Autodesk Inventor part; units mm, degrees
ref_plane "YZ Plane" through (0, 0, 0) normal (1, 0, 0) x (0, 1, 0)
ref_plane "XZ Plane" through (0, 0, 0) normal (0, 1, 0) x (-1, 0, 0)
ref_plane "XY Plane" through (0, 0, 0) normal (0, 0, 1) x (1, 0, 0)
sketch "Эскиз1" plane through (0, 0, 0) normal (0, 0, 1) x (1, 0, 0)
  line L0 (0, 81) -> (0, 93)
  line L1 (0, 93) -> (-11, 93)
  line L2 (-11, 93) -> (-11, 81.2677)
  line L3 (-11, 81.2677) -> (-42, 50)
  line L4 (-42, 50) -> (-42, 26)
  line L5 (-42, 26) -> (-38, 26)
  line L6 (-38, 26) -> (-38, 42.6719)
  line L7 (-38, 42.6719) -> (0, 81)
  line L8 (0, 0) -> (0, 108.7974) construction
  line L9 (-50.4, 0) -> (8.4, 0)
  dimension "d0" = 11
  dimension "d1" = 12
  dimension "d2" = 24
  dimension "d3" = 4
  dimension "d4" = 8
  dimension "d5" = 67
  dimension "d6" = 42
  dimension "d7" = 93
revolve "Вращение1" add sketch "Эскиз1" angle 360 about axis through (-10, 0, 0) along (1, 0, 0)
hole "Отверстие1" at (-11, -0.0233, 87.0155) direction (1, 0, 0) diameter 5 end through all counterbore diameter 9 counterbore depth 5
pattern_circular "Круговой массив1" count 6 over 360 about axis through (-10, 0, 0) along (1, 0, 0) of "Отверстие1"
CAD build for the part. Positions are in the model's coordinates, mm. A direction names the side the tool comes from. Round coordinates to 2 decimals unless told otherwise and drop trailing zeros. Write each loop counter-clockwise with the first axis right and the second up, starting at its lowest first coordinate (ties: lowest second). Pieces come first, ordered by that corner, then holes. Notation, with made-up numbers: M -36.75,65.5 L -8.75,65.5 A16 ccw -8.75,92.5 Z; hole C 7.25,72.5 d2. An arc over 180 degrees is marked long. Put each result on its own line as item: value. Start each with the question number.
1) 3-axis set-ups, long thin cutter, end or side, ignore diameter. For faces 1 (the cylindrical face through (-2.958, -77.825, -43.853)), 2 (the flat face through (-6, -2, -89)): which of +Z, -Z, +X, -X, +Y, -Y reach the whole face in a straight line?
2) Saw through at A-A, the plane z = 0. Write the cut outline in (x, y), and give its area (3 significant figures).
3) Pin check, flat tips, straight feed: pin 1 Ø2.5 at (y, z) = (76, -44.5) entering from -X; pin 2 Ø2 at (x, y) = (-14.5, -11.5) entering from +Z; pin 3 Ø5 at (x, z) = (-20, -29.5) entering from -Y; pin 4 Ø10.5 at (y, z) = (-75.35, -43.53) entering from -X. Stop position of each tip, or through.
4) Drill centre lines: probe 1 along Y at (x, z) = (-10, -40.5); probe 2 along Z at (x, y) = (-8, -14); probe 3 along Y at (x, z) = (-5.5, 33.5). Where is each one in solid material? Low to high. Write a range as [from, to].
5) Saw through at C-C, the plane x = -33.5. Write the cut outline in (y, z).
6) Saw through at B-B, the plane x = -21. Write the cut outline in (y, z).
7) Pull direction Y, two halves, no side cores. Call faces 3 (the flat face through (-38, -20, -18)), 4 (the conical face through (-40.06, -11.26, -50.72)), 5 (the flat face through (0, -28, 76.2)): pulls with the +Y half, pulls with the -Y half, needs draft (parallel to the pull), parting line crosses it, or undercut.
Resolved:
1. face 1: +X, -X
1. face 2: -X
2. outline: M -42,-50 L -11,-81.27 L -11,-93 L 0,-93 L 0,-81 L -38,-42.67 L -38,-26 L -42,-26 Z; M -42,26 L -38,26 L -38,42.67 L 0,81 L 0,93 L -11,93 L -11,81.27 L -42,50 Z
2. area: 1,210 mm²
3. pin 1: through
3. pin 2: z = 77.91
3. pin 3: y = -68.84
3. pin 4: x = -11
4. probe 1: [-83.72, -78.67], [-72.02, -58.21], [58.21, 72], [78.73, 83.72]
4. probe 2: [-91.94, -71.57], [71.57, 91.94]
4. probe 3: [-86.76, -67.61], [67.61, 86.76]
5. outline: C 0,0 d117.15; hole C 0,0 d94.42
6. outline: C 0,0 d142.36; hole C 0,0 d119.64
7. face 3: undercut
7. face 4: parting line crosses it
7. face 5: needs draft
